Print and shaded views of the part. All mm, measured from the part's lowest x, y and z. A direction names the side the tool comes from. Coordinates: 2 decimals unless noted, no trailing zeros. Order: outer loops, then holes, each group sorted by start corner. A loop starts at its lowest first (then second) coordinate and runs counter-clockwise, first axis right, second up. Notation, with made-up numbers: M -17,14 L 40,14 A9 ccw 40,25 Z; hole C 85,74.25 d6. An arc over 180 degrees is marked long. Return JSON: item names as keys, results as strings.
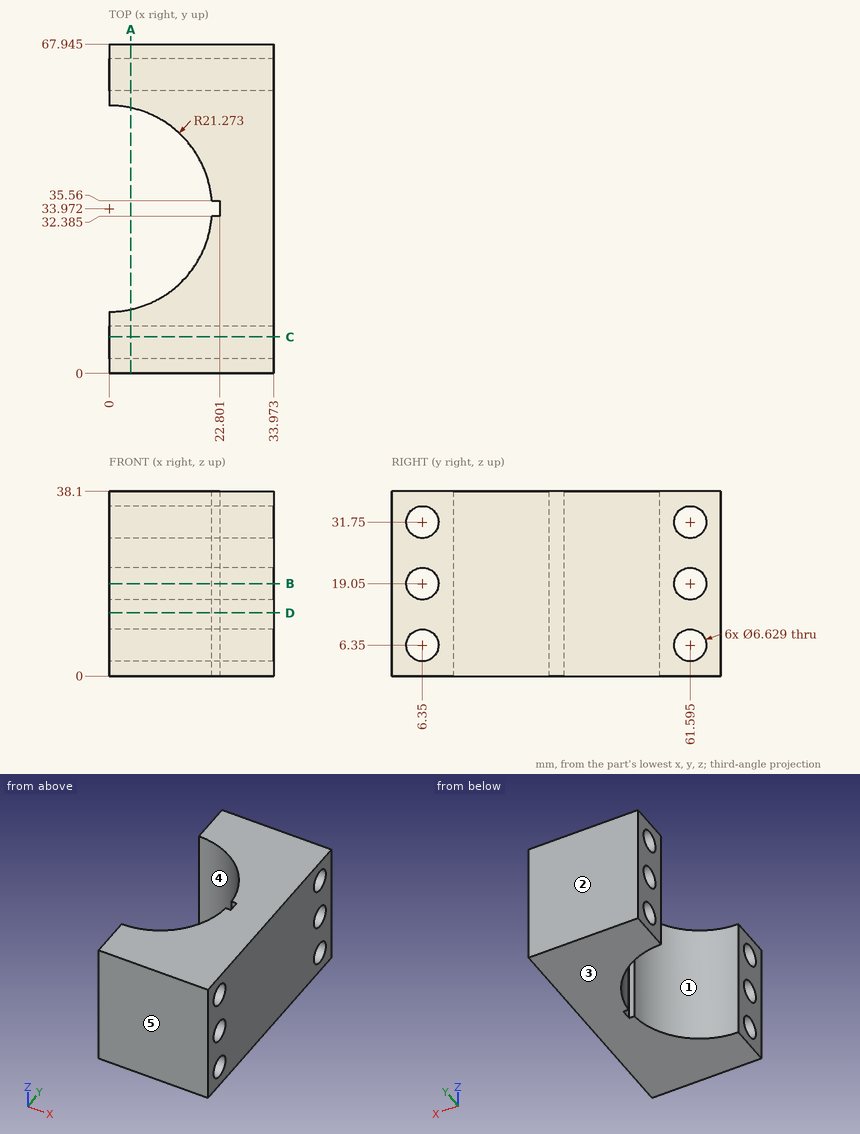
Item 1: Saw through at B-B (z = 19.05). Write the cut outline in (x, y) (1 decimal).
Check result:
{"outline": "M 0,0 L 34,0 L 34,3 L 0,3 Z; M 0,9.7 L 34,9.7 L 34,58.3 L 0,58.3 L 0,55.2 A21.3 cw 21.2,35.6 L 22.8,35.6 L 22.8,32.4 L 21.2,32.4 A21.3 cw 0,12.7 Z; M 0,64.9 L 34,64.9 L 34,67.9 L 0,67.9 Z"}
Item 2: Pull direction Y, two halves, no side cores. Call the marked faces 1, 2 and 3: +Y half, -Y half, draft (parallel to the pull), parting line (faces both ways), or undercut.
Check result:
{"face 1": "undercut", "face 2": "+Y half", "face 3": "draft"}
Item 3: Saw through at D-D (z = 13). Write the cut outline in (x, y) (1 decimal), and give its area (3 significant figures).
Check result:
{"outline": "M 0,0 L 34,0 L 34,67.9 L 0,67.9 L 0,55.2 A21.3 cw 21.2,35.6 L 22.8,35.6 L 22.8,32.4 L 21.2,32.4 A21.3 cw 0,12.7 Z", "area": "1,590 mm2"}
Item 4: 3-axis set-ups, long thin cutter, end or side, ignore diameter. For the marked faces 4 and 5: which of +Z, -Z, +X, -X, +Y, -Y reach the whole face in a straight line?
Check result:
{"face 4": "+Z, -Z, -X", "face 5": "+Z, -Z, +X, -X, -Y"}
Item 5: Wall check: line 1 (Y direction, x = 22, z = 31.75) (1 decimal); line 2 (Y direction, x = 18.5, z = 6.35) (1 decimal); line 3 (Z direction, x = 7.5, y = 64). Give the ranges that are in metal, low to high.
Check result:
{"line 1": "y = 0 to 3, 9.7 to 32.4, 35.6 to 58.3, 64.9 to 67.9", "line 2": "y = 0 to 3, 9.7 to 23.5, 44.5 to 58.3, 64.9 to 67.9", "line 3": "z = 0 to 4.07, 8.63 to 16.77, 21.33 to 29.47, 34.03 to 38.1"}
Item 6: Saw through at C-C (y = 7.5). Write the cut outline in (x, z).
Check result:
{"outline": "M 0,0 L 33.97,0 L 33.97,3.24 L 0,3.24 Z; M 0,9.46 L 33.97,9.46 L 33.97,15.94 L 0,15.94 Z; M 0,22.16 L 33.97,22.16 L 33.97,28.64 L 0,28.64 Z; M 0,34.86 L 33.97,34.86 L 33.97,38.1 L 0,38.1 Z"}
Item 7: Drop flat-ended pins along their axis: pin 1 Ø6 at (y, z) = (28.5, 28.5) entering from -X; pin 2 Ø4 at (y, z) = (32, 17.5) entering from -X; pin 3 Ø1 at (y, z) = (34, 23.5) entering from -X. Give the stop position or say it passes through.
Check result:
{"pin 1": "stops at x = 19.51", "pin 2": "stops at x = 20.9", "pin 3": "stops at x = 22.8"}
Item 8: Saw through at A-A (x = 4.5). Count the separate pieces of the cut face and the enclosed holes in it.
Check result:
{"separate pieces": "2", "enclosed holes": "6"}
